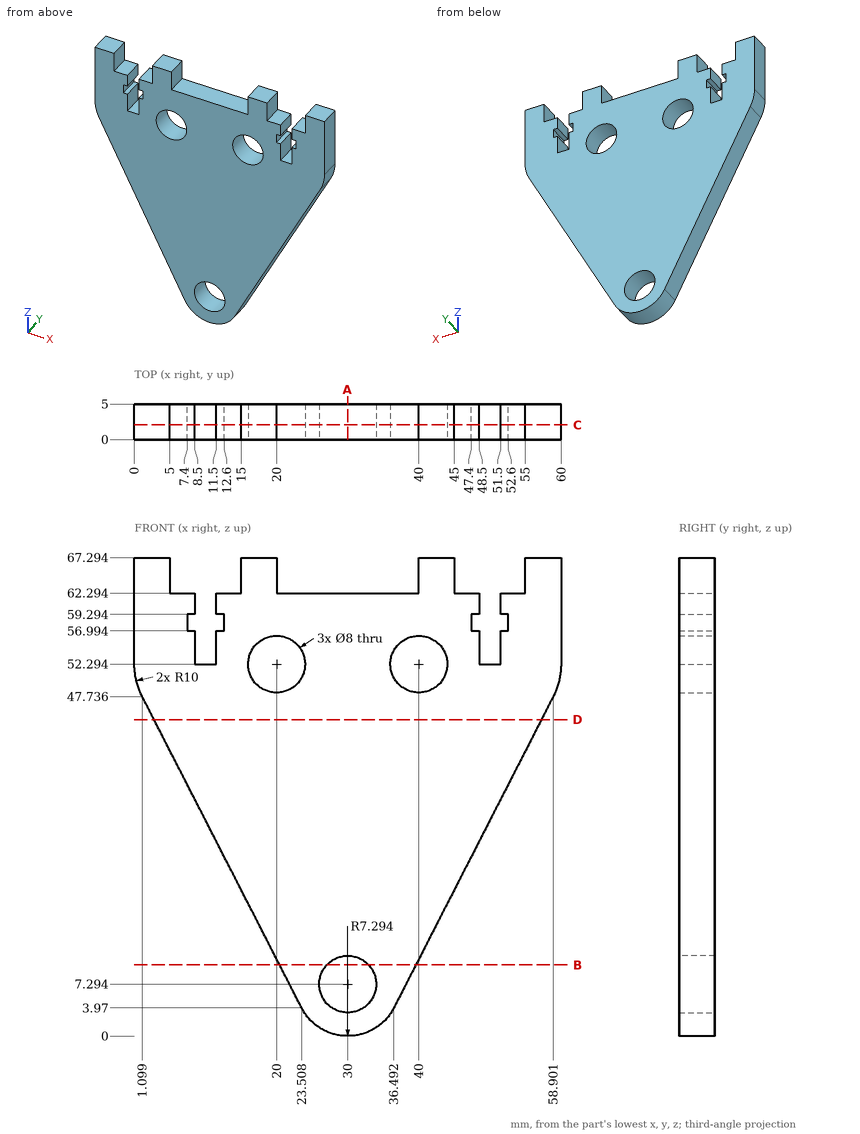
Source: three-view drawing plus pictorial views. Frame: mm from the lowest corner of the part. Coordinates: 2 decimals unless noted, no trailing zeros. Write each loop counter-clockwise with the first axis right and the second up, starting at its lowest first coordinate (ties: lowest second). Pieces come first, ordered by that corner, then holes. Notation, with made-up numbers: (-13.5, 35.25) -> (19.5, 35.25) arc R30 ccw to (19.5, 58.25) -> close; hole circle Ø10 at (-20, 64.5). An arc over 180 degrees is marked (long way). Answer as a JSON object with one key per item and string values.
1. Section A-A on x = 30. Return the cut outline in (y, z).
Result set:
{"outline": "(0, 0) -> (5, 0) -> (5, 3.29) -> (0, 3.29) -> close; (0, 11.29) -> (5, 11.29) -> (5, 62.29) -> (0, 62.29) -> close"}
2. Section D-D on z = 44.5. Return the cut outline in (x, y).
Result set:
{"outline": "(2.76, 0) -> (57.24, 0) -> (57.24, 5) -> (2.76, 5) -> close"}
3. Section B-B on z = 10. Return the cut outline in (x, y) (1 decimal).
Result set:
{"outline": "(20.4, 0) -> (27.1, 0) -> (27.1, 5) -> (20.4, 5) -> close; (32.9, 0) -> (39.6, 0) -> (39.6, 5) -> (32.9, 5) -> close"}
4. First-contact query: P1, Ø0.6, axis at x = 52, y = 3.5, coming from the +Z side; P2, Ø0.9, axis at x = 12, y = 3.5, coming from the -Z side (1 decimal); P3, Ø1.5, axis at y = 2.5, z = 10, coming from the +X side. Flat tips, straight axial feed; report the tip coordinate or a pass-through.
Result set:
{"P1": "stops at z = 62.29", "P2": "stops at z = 25.6", "P3": "stops at x = 39.96"}
5. Section C-C on y = 2.05. Count the separate pieces of the cut face and the enclosed holes in it, then the cut area to 4 significant figures.
Result set:
{"separate pieces": "1", "enclosed holes": "3", "area": "2,335 mm2"}
6. Material intervals for line 1 (X direction, y = 3.5, z = 63); line 2 (Z direction, x = 22.5, y = 2.9) (1 decimal); line 3 (X direction, y = 4.6, z = 10) (1 decimal), sorted ascending. Write a range as from..to.
Result set:
{"line 1": "x = 0..5, 15..20, 40..45, 55..60", "line 2": "z = 5.9..49.2, 55.4..62.3", "line 3": "x = 20.4..27.1, 32.9..39.6"}
